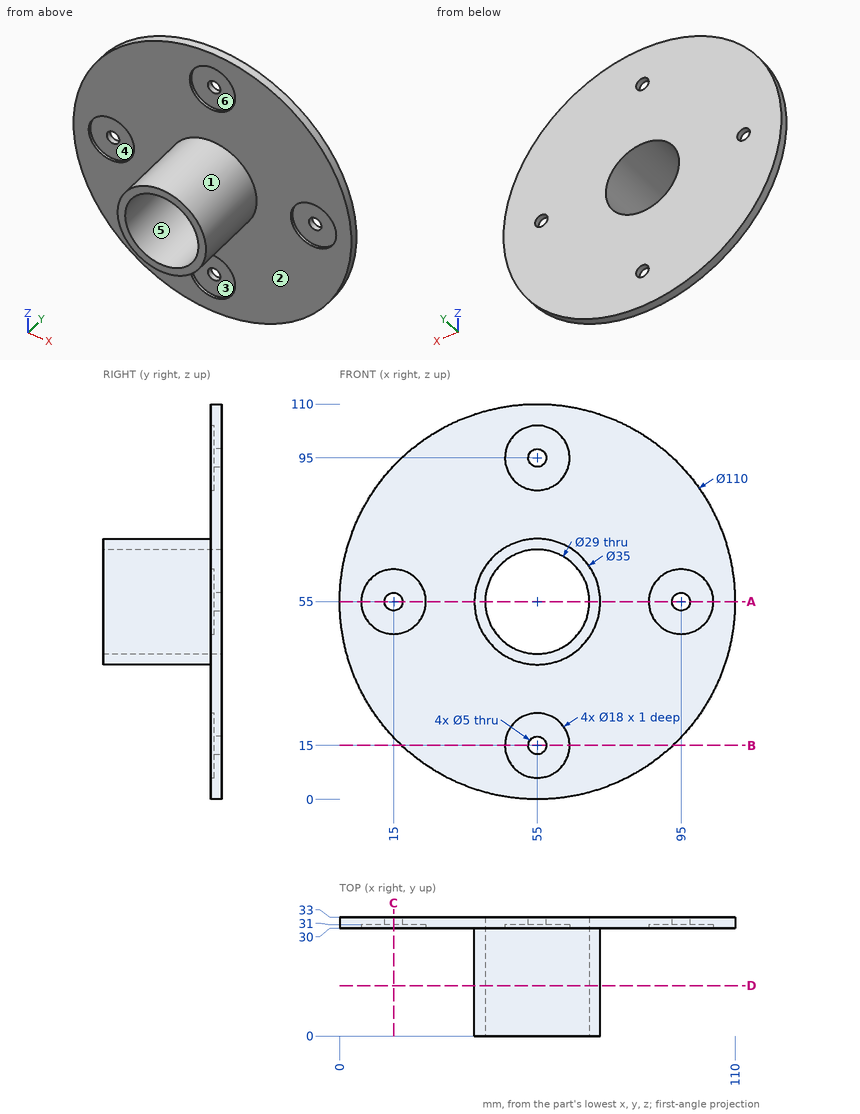
Geometry check sheet. Reference: drawing and pictorial views, mm from the part's lowest x, y, z. A direction names the side the tool comes from. Give positions to 0.01 mm unless a question says otherwise; leave off trailing zeros. Loops run counter-clockwise (first coordinate to the right, second up) from the corner with the lowest first, then second, coordinate; pieces in that order, holes last. Notation, with made-up numbers: M -34,-32.75 L 18,-32.75 A32 ccw 18,-0.75 Z; hole C 81,28.5 d3. An arc over 180 degrees is marked long. Use a Markdown table: item, result. Add a question column.
Q1. Sectioned sample at C-C, the plane x = 15. Record the cut outline in (y, z), then the cut area to 3 significant figures.
Q2. Scan lines: line 1 along X through (y, z) = (32.35, 55); line 2 along Y through (x, z) = (67, 18); line 3 along Y through (x, z) = (98, 58.5). Record each from-to range of solid material in increasing order. Write a range as [from, to].
Q3. Sectioned sample at D-D, the plane y = 14. Record the cut outline in (x, z).
Q4. Tool access check on the marked faces 5 and 6. Record the directions out of +Z, -Z, +X, -X, +Y, -Y that give a thin tool (end or side, any length) a straight path to the whole face; none if there is none.
Q5. Sectioned sample at A-A, the plane z = 55. Record the cut outline in (x, y).
Q6. Mould release check, pull along X, two halves, no side actions. Record for the marked faces 1, 2, 3 and 4: pulls with the +X half, pulls with the -X half, needs draft (parallel to the pull), parting line crosses it, or undercut.
Q7. Go/stop test with flat-tipped pins: pin 1 (5.5 mm diameter, centred on x = 58.5, z = 17.5, fed in from -Y); pin 2 (2 mm diameter, centred on x = 64, y = 21.5, fed in from +Z); pin 3 (23.5 mm diameter, centred on x = 55, z = 15, fed in from -Y); pin 4 (20.5 mm diameter, centred on x = 95, z = 55, fed in from +Y). Record where each tip stops, or that it passes through.
Q8. Sectioned sample at B-B, the plane z = 15. Record the cut outline in (x, y), then the cut area to 3 significant figures.
Verdict:
| question | item | result |
|---|---|---|
| 1 | outline | M 30,17.25 L 33,17.25 L 33,52.5 L 31,52.5 L 31,46 L 30,46 Z; M 30,64 L 31,64 L 31,57.5 L 33,57.5 L 33,92.75 L 30,92.75 Z |
| 1 | area | 198 mm^2 |
| 2 | line 1 | [0, 12.5], [17.5, 40.5], [69.5, 92.5], [97.5, 110] |
| 2 | line 2 | [30, 33] |
| 2 | line 3 | [31, 33] |
| 3 | outline | C 55,55 d35; hole C 55,55 d29 |
| 4 | face 5 | +Y, -Y |
| 4 | face 6 | -Y |
| 5 | outline | M 0,30 L 6,30 L 6,31 L 12.5,31 L 12.5,33 L 0,33 Z; M 17.5,31 L 24,31 L 24,30 L 37.5,30 L 37.5,0 L 40.5,0 L 40.5,33 L 17.5,33 Z; M 69.5,0 L 72.5,0 L 72.5,30 L 86,30 L 86,31 L 92.5,31 L 92.5,33 L 69.5,33 Z; M 97.5,31 L 104,31 L 104,30 L 110,30 L 110,33 L 97.5,33 Z |
| 6 | face 1 | parting line crosses it |
| 6 | face 2 | needs draft |
| 6 | face 3 | undercut |
| 6 | face 4 | undercut |
| 7 | pin 1 | y = 31 |
| 7 | pin 2 | z = 70.56 |
| 7 | pin 3 | y = 30 |
| 7 | pin 4 | y = 33 |
| 8 | outline | M 17.25,30 L 46,30 L 46,31 L 52.5,31 L 52.5,33 L 17.25,33 Z; M 57.5,31 L 64,31 L 64,30 L 92.75,30 L 92.75,33 L 57.5,33 Z |
| 8 | area | 198 mm^2 |
